Design review of the part shown in the three views and the two pictorial views. Dimensions are in mm from the part's minimum x, y and z. A direction names the side the tool comes from. Coordinates: 2 decimals unless noted, no trailing zeros. Loops run counter-clockwise (first coordinate to the right, second up) from the corner with the lowest first, then second, coordinate; pieces in that order, holes last.
Q1. Add section D-D on x = 120. Give the boundary of the cut face in (y, z), and give its area (3 significant figures).
Q2. Wall thickness on probe 1 along X at (y, z) = (194.75, 150); probe 2 along Y at (x, z) = (118.5, 121.5); probe 3 along X at (y, z) = (220, 71.5): over which ranges is each line inside the solid? List them lowest first.
Q3. Add section C-C on z = 150. Give the boundary of the cut face in (x, y).
Q4. For P1, Ø8, axis at x = 221, z = 104, coming from the -Y side; P2, Ø8, axis at x = 240.5, z = 210, coming from the -Y side; P3, Ø12, axis at x = 249, y = 266, coming from the +Z side, all flat-tipped, find the tip position at first contact; note any pin that passes through.
Q5. Add section B-B on y = 150. Give the boundary of the cut face in (x, z), and give its area (3 significant figures).
Q6. Draft analysis for pull direction Y (two halves, no side actions). For the marked faces 5, 6, 7 and 8, state which applies: released by +Y, released by -Y, zero draft, split by the parting line, or undercut.
Q7. Machinability: for the marked faces 1, 2, 3 and 4, which of the approach directions +Z, -Z, +X, -X, +Y, -Y give a long, thin tool a straight path to every point of the face, cutting with its end or side? Answer none if there is none.
Q8. Add section A-A on x = 50. Give the boundary of the cut face in (y, z).
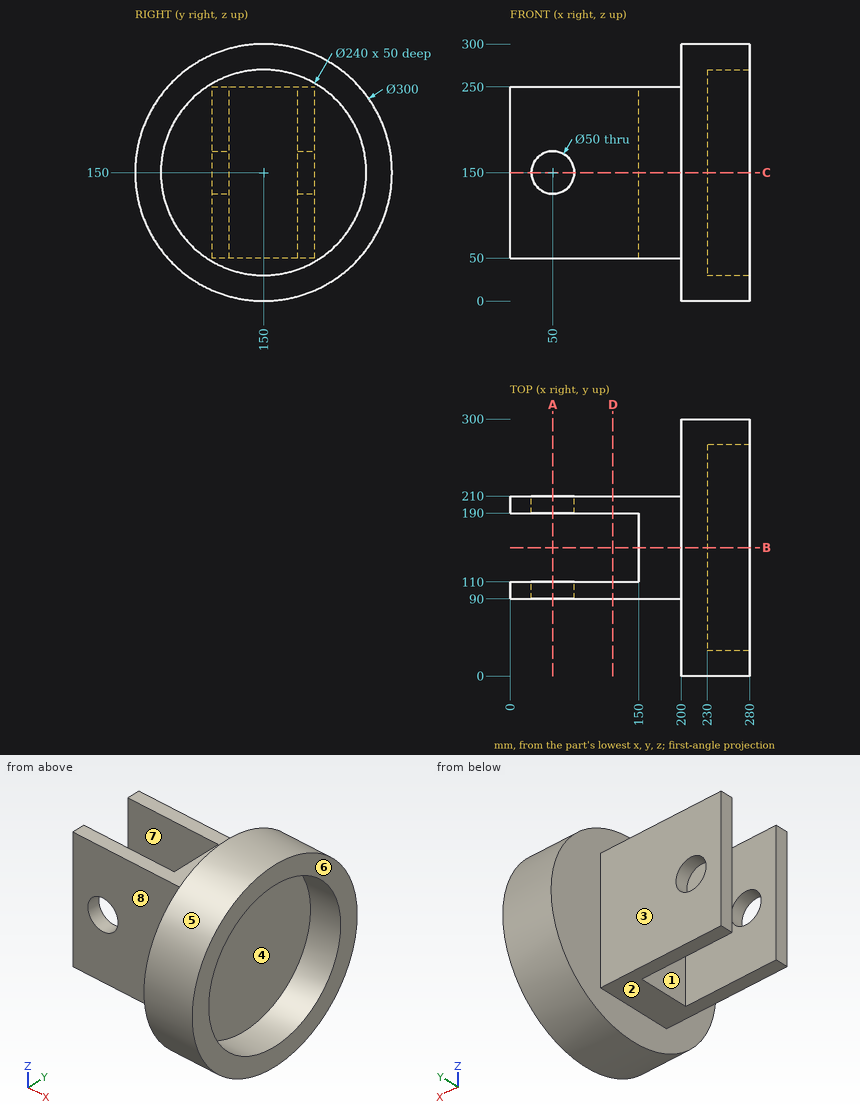
Entries:
1. outline: (90, 50) - (110, 50) - (110, 250) - (90, 250) - close; (190, 50) - (210, 50) - (210, 250) - (190, 250) - close
1. area: 8,000 mm2
2. probe 1: x = 0 to 25, 75 to 230
2. probe 2: y = 90 to 110, 190 to 210
2. probe 3: x = 200 to 230
3. outline: (0, 90) - (25, 90) - (25, 110) - (0, 110) - close; (0, 190) - (25, 190) - (25, 210) - (0, 210) - close; (75, 90) - (200, 90) - (200, 0) - (280, 0) - (280, 30) - (230, 30) - (230, 270) - (280, 270) - (280, 300) - (200, 300) - (200, 210) - (75, 210) - (75, 190) - (150, 190) - (150, 110) - (75, 110) - close
4. P1: stops at y = 6
4. P2: stops at y = 10.85
4. P3: stops at z = 251.98
5. outline: (150, 50) - (200, 50) - (200, 0) - (280, 0) - (280, 30) - (230, 30) - (230, 270) - (280, 270) - (280, 300) - (200, 300) - (200, 250) - (150, 250) - close
5. area: 22,000 mm2
6. face 5: split by the parting line
6. face 6: zero draft
6. face 7: undercut
6. face 8: released by -Y
7. face 1: +Z, -Z, -X
7. face 2: -Z, -X, +Y, -Y
7. face 3: +Z, -Z, -X, +Y
7. face 4: +X
8. outline: (90, 50) - (110, 50) - (110, 125) - (90, 125) - close; (90, 175) - (110, 175) - (110, 250) - (90, 250) - close; (190, 50) - (210, 50) - (210, 125) - (190, 125) - close; (190, 175) - (210, 175) - (210, 250) - (190, 250) - close
